Check sheet for the drawn part. Datum: minimum x, y, z corner. Units: mm. Give positions to 0.01 mm unless a question says otherwise; leave off trailing zeros. Loops run counter-clockwise (first coordinate to the right, second up) from the corner with the lowest first, then second, coordinate; pieces in that order, holes last. Notation, with made-up numbers: (65, -16.75) - (103, -16.75) arc R33 cw to (103, 18.25) - close; hole circle Ø8 at (81.25, 64). An arc over 180 degrees is marked (long way). Use one line per item in the form item = value.
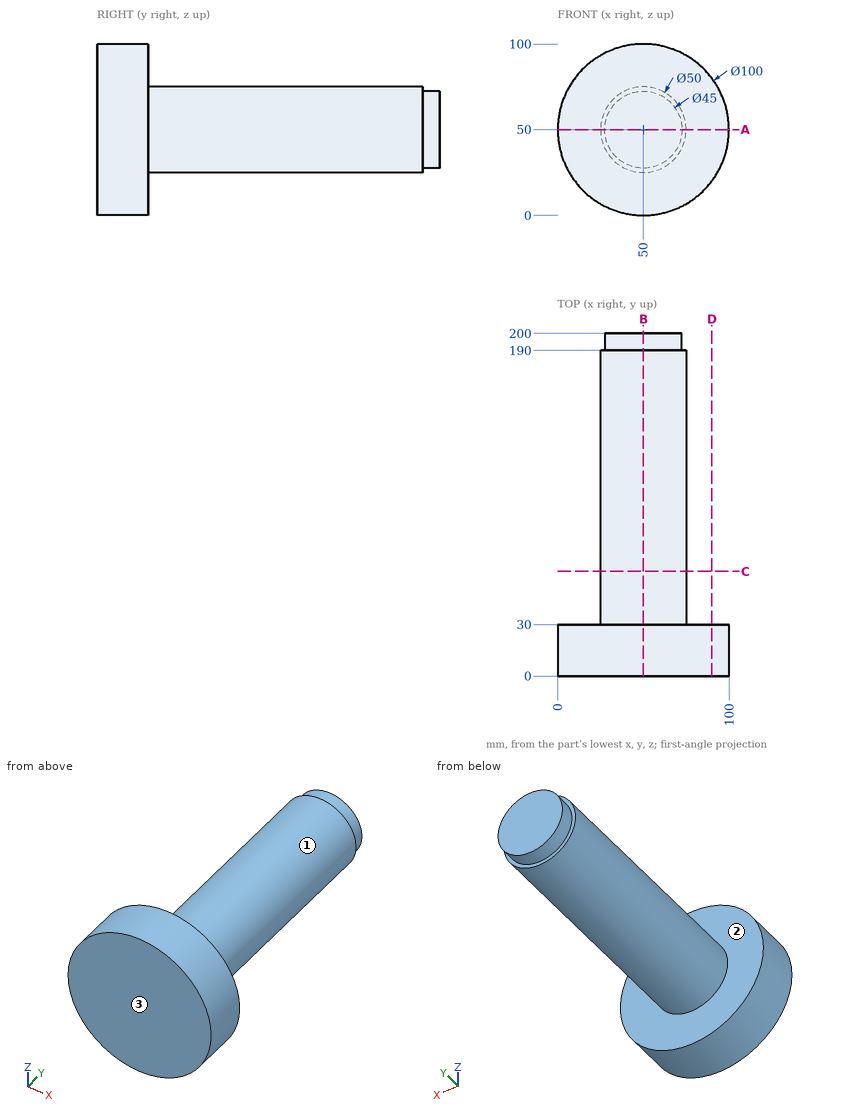
1. Section check B-B, the plane x = 50. Record the cut outline in (y, z), then the cut area to 4 significant figures.
Result set:
outline = (0, 0) - (30, 0) - (30, 25) - (190, 25) - (190, 27.5) - (200, 27.5) - (200, 72.5) - (190, 72.5) - (190, 75) - (30, 75) - (30, 100) - (0, 100) - close
area = 11,450 mm²
2. Section check A-A, the plane z = 50. Record the cut outline in (x, y), then the cut area to 4 significant figures.
Result set:
outline = (0, 0) - (100, 0) - (100, 30) - (75, 30) - (75, 190) - (72.5, 190) - (72.5, 200) - (27.5, 200) - (27.5, 190) - (25, 190) - (25, 30) - (0, 30) - close
area = 11,450 mm²
3. Draft check along Y on the marked faces 1, 2 and 3. Enter one of: released by +Y, released by -Y, zero draft, split by the parting line, or undercut.
Result set:
face_1 = zero draft
face_2 = released by +Y
face_3 = released by -Y
4. Section check C-C, the plane y = 61. Record the cut outline in (x, z), then the cut area to 3 significant figures.
Result set:
outline = circle Ø50 at (50, 50)
area = 1,960 mm²
5. Section check D-D, the plane x = 90. Record the cut outline in (y, z).
Result set:
outline = (0, 20) - (30, 20) - (30, 80) - (0, 80) - close
6. Scan lines: probe 1 along Z at (x, y) = (50, 20); probe 2 along Y at (x, z) = (28, 66.5); probe 3 along Y at (x, z) = (55.5, 26.5). Record each from-to range of solid material in increasing order.
Result set:
probe_1 = 0 to 100
probe_2 = 0 to 30
probe_3 = 0 to 190
7. Depth check by flat-ended pin: pin 1 Ø12 at (y, z) = (135, 57) entering from -X; pin 2 Ø3 at (x, y) = (60.5, 80.5) entering from -Z; pin 3 Ø6 at (x, y) = (71.5, 100.5) entering from -Z. Enter the tip coordinate at first touch or a pass-through.
Result set:
pin_1 = 25.02
pin_2 = 26.68
pin_3 = 33.18
